from build123d import *

# Parameters (mm, degrees)
CROQUIS1_R              = 15
SALIENTE_EXTRUIR1_DEPTH = 3
CROQUIS3_R              = 9
SALIENTE_EXTRUIR3_DEPTH = 58
SALIENTE_EXTRUIR4_START = 3
CROQUIS4_R              = 15
SALIENTE_EXTRUIR4_DEPTH = 3
CORTAR_EXTRUIR1_DEPTH   = 8
CROQUIS8_R              = 12.5
CROQUIS8_R_2            = 9
SALIENTE_EXTRUIR7_DEPTH = 58
REDONDEO3_R             = 5
CORTAR_EXTRUIR2_DEPTH   = 40


with BuildPart() as part:
    # Croquis1 → Saliente-Extruir1 (new body)
    with BuildSketch(Plane.XY):
        Circle(CROQUIS1_R)
    extrude(amount=SALIENTE_EXTRUIR1_DEPTH)

    # Croquis3 → Saliente-Extruir3 (add)
    with BuildSketch(Plane(origin=(0, 0, 0), x_dir=(-1, 0, 0), z_dir=(0, 0, -1))):
        with Locations(Location((0, 0, 0), (0, 0, 180))):
            Circle(CROQUIS3_R)
    extrude(amount=SALIENTE_EXTRUIR3_DEPTH)

    # Croquis4 → Saliente-Extruir4 (add)
    with BuildSketch(Plane(origin=(0, 0, -58), x_dir=(-1, 0, 0), z_dir=(0, 0, -1)).offset(SALIENTE_EXTRUIR4_START)):
        with Locations(Location((0, 0, 0), (0, 0, 180))):
            Circle(CROQUIS4_R)
    extrude(amount=-SALIENTE_EXTRUIR4_DEPTH)

    # Croquis5 → Cortar-Extruir1 (cut)
    with BuildSketch(Plane(origin=(0, 0, -61), x_dir=(-1, 0, 0), z_dir=(0, 0, -1))):
        with BuildLine():
            Line((2.045621727, 0.133909486), (-0.160815889, 2.043682522))
            ThreePointArc((-0.160815889, 2.043682522), (-1.341615267, -1.550022089), (2.045621727, 0.133909486))
        make_face()
    extrude(amount=-CORTAR_EXTRUIR1_DEPTH, mode=Mode.SUBTRACT)

    # Croquis8 → Saliente-Extruir7 (add)
    with BuildSketch(Plane(origin=(0, 0, 0), x_dir=(-1, 0, 0), z_dir=(0, 0, -1))):
        with Locations(Location((0, 0, 0), (0, 0, 180))):
            Circle(CROQUIS8_R)
        Circle(CROQUIS8_R_2, mode=Mode.SUBTRACT)
    extrude(amount=SALIENTE_EXTRUIR7_DEPTH)

    # Redondeo3
    # the kernel refuses this fillet: 5 mm, written as the material it adds along each edge
    with BuildSketch(Plane(origin=(0, 0, -58), x_dir=(1, 0, 0), z_dir=(0, 1, 0))) as redondeo3_piece_1:
        with BuildLine():
            CenterArc((17.5, -4.330127019), REDONDEO3_R, 120, 60)
            Line((12.5, -4.330127019), (12.4, -4.330127019))
            Line((12.4, -4.330127019), (12.4, 0))
            Line((12.4, 0), (12.5, 0.1))
            ThreePointArc((12.5, 0.1), (13.75, 0.1), (14.95, 0.08660254))
            Line((14.95, 0.08660254), (15, 0))
        make_face()
    revolve(axis=Axis((0, 0, -58), (0, 0, -1)))
    with BuildSketch(Plane(origin=(0, 0, 0), x_dir=(1, 0, 0), z_dir=(0, 1, 0))) as redondeo3_piece_2:
        with BuildLine():
            CenterArc((17.5, 4.330127019), REDONDEO3_R, 180, 60)
            Line((15, 0), (14.95, -0.08660254))
            ThreePointArc((14.95, -0.08660254), (13.75, -0.1), (12.5, -0.1))
            Line((12.5, -0.1), (12.4, 0))
            Line((12.4, 0), (12.4, 4.330127019))
            Line((12.4, 4.330127019), (12.5, 4.330127019))
        make_face()
    revolve(axis=Axis((0, 0, 0), (0, 0, -1)))

    # Croquis2 → Cortar-Extruir2 (cut)
    with BuildSketch(Plane.XY.offset(3)):
        Polygon((3.013979252, -2.718374956), (3.861171395, 1.250995121), (0.847192143, 3.969370077), (-3.013979252, 2.718374956), (-3.861171395, -1.250995121), (-0.847192143, -3.969370077), align=None)
    extrude(amount=-CORTAR_EXTRUIR2_DEPTH, mode=Mode.SUBTRACT)


solid = part.part
Model file for the job. Use its own axes, mm. A direction names the side the tool comes from. Give positions to 0.01 mm unless a question says otherwise; leave off trailing zeros. Order: outer loops, then holes, each group sorted by start corner. A loop starts at its lowest first (then second) coordinate and runs counter-clockwise, first axis right, second up. Notation, with made-up numbers: (35, 22) - (91, 22) arc R28 ccw to (91, 44) - close; hole circle Ø4 at (86, 5). An arc over 180 degrees is marked (long way). Return JSON: item names as keys, results as strings.
1) Flat gauge pins, fed straight in: P1, Ø5, axis at y = 11, z = -27.5, coming from the +X side; P2, Ø3, axis at y = -9, z = -34, coming from the -X side; P3, Ø1, axis at y = 1, z = -48.5, coming from the +X side. Where does each tip first touch, or does it go through?
Geometry says:
{"P1": "x = 9.17", "P2": "x = -10", "P3": "x = 12.49"}
2) Cut at A-A, the plane z = -15. Give the cut face in (x, y).
Geometry says:
{"outline": "circle Ø25 at (0, 0); hole (-3.86, -1.25) - (-0.85, -3.97) - (3.01, -2.72) - (3.86, 1.25) - (0.85, 3.97) - (-3.01, 2.72) - close"}
3) 3-axis set-ups, long thin cutter, end or side, ignore diameter. For faces 4 (the flat face through (-0.958, 1.075, -57.056)), 5 (the flat face through (-1.06, 3.35, -16.72)), 6 (the cylindrical face through (8.06, -12.65, -59.52)): which of +Z, -Z, +X, -X, +Y, -Y reach the whole face in a straight line?
Geometry says:
{"face 4": "-Z", "face 5": "+Z", "face 6": "+Z, -Z"}
4) Probe line 1 (X direction, y = 0, z = -55); line 2 (Y direction, x = 0, z = -57.25); line 3 (Z direction, x = -6, y = -12). List the from-to ranges inside material, lowest first. Write a range as from..to.
Geometry says:
{"line 1": "-12.68..-2.05, 2.05..12.68", "line 2": "-14.01..-2.05, 1.9..14.01", "line 3": "-61..-56.56, -1.44..3"}
5) Pull direction X, two halves, no side cores. Call faces 1 (the flat face through (3, -3, 3)), 2 (the flat face through (0, 0, -53)), 3 (the cylindrical face through (11.923, -3.755, -28.655)): pulls with the +X half, pulls with the -X half, needs draft (parallel to the pull), parting line crosses it, or undercut.
Geometry says:
{"face 1": "needs draft", "face 2": "undercut", "face 3": "parting line crosses it"}
6) Cut at B-B, the plane z = -47.5. Give the cut face in (x, y).
Geometry says:
{"outline": "circle Ø25 at (0, 0)"}
